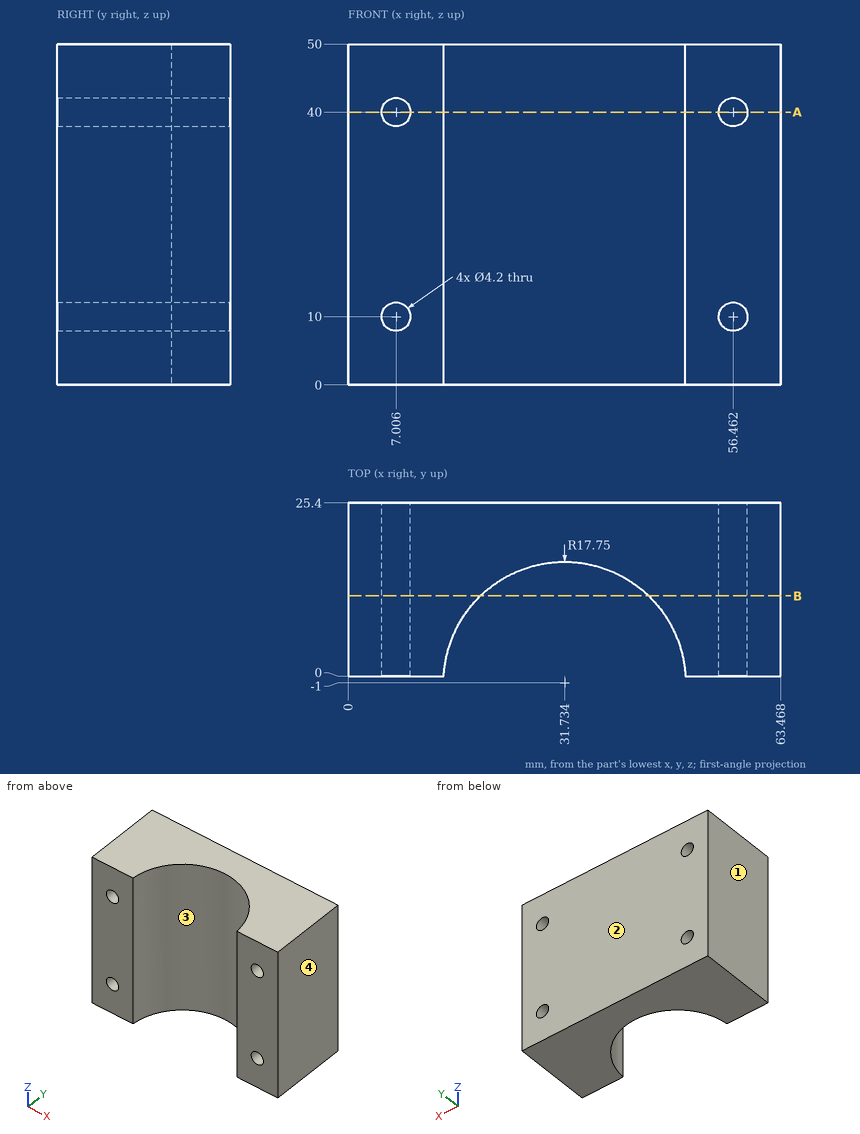
For this review, use the dimensioned drawing (mm, ordinates from the lowest corner) and the shaded views. Round coordinates to 2 decimals unless told otherwise and drop trailing zeros. Order: outer loops, then holes, each group sorted by start corner. A loop starts at its lowest first (then second) coordinate and runs counter-clockwise, first axis right, second up. Notation, with made-up numbers: (-10.75, 20) -> (-2.75, 20) arc R31 ccw to (-2.75, 54) -> close; hole circle Ø1 at (5.5, -40). An arc over 180 degrees is marked (long way). Write item = value, one per line. Start each with the question number.
Item 1: Mouldability with a two-part tool opening along X and no side actions: class the marked faces 1, 2, 3 and 4 as released by +X, released by -X, zero draft, split by the parting line, or undercut.
Item 2: Consider section A-A on z = 40. Count the separate pieces of the cut face and the enclosed holes in it.
Item 3: Consider section B-B on y = 11.75. Write out the cut boundary in (x, z) (1 decimal).
Item 4: For line 1 along Z through (x, y) = (8, 20); line 2 along X through (y, z) = (17.75, 40); line 3 along X through (y, z) = (13.5, 10) (1 decimal), list the stretches that pass through material, from the lowest coordinate up.
Conclusion:
q1.face_1 = released by -X
q1.face_2 = zero draft
q1.face_3 = undercut
q1.face_4 = released by +X
q2.separate_pieces = 3
q2.enclosed_holes = 0
q3.outline = (0, 0) -> (19.4, 0) -> (19.4, 50) -> (0, 50) -> close; (44.1, 0) -> (63.5, 0) -> (63.5, 50) -> (44.1, 50) -> close; hole circle Ø4.2 at (7, 10); hole circle Ø4.2 at (7, 40); hole circle Ø4.2 at (56.5, 10); hole circle Ø4.2 at (56.5, 40)
q4.line_1 = 0 to 8.15, 11.85 to 38.15, 41.85 to 50
q4.line_2 = 0 to 4.91, 9.11 to 54.36, 58.56 to 63.47
q4.line_3 = 0 to 4.9, 9.1 to 21.5, 42 to 54.4, 58.6 to 63.5
